Autodesk Inventor part; units mm, degrees
ref_plane "to_cp1_XY" through (0, 0, 0) normal (1, 0, 0) x (0, 0, -1)
ref_plane "to_cp1_YZ" through (0, 0, 0) normal (0, 0, -1) x (0, 1, 0)
ref_plane "to_cp1_ZX" through (0, 0, 0) normal (0, 1, 0) x (1, 0, 0)
sketch "Sketch_1" plane through (0, 0, 0) normal (0, 0, 1) x (1, 0, 0)
  line L0 (50, 0) -> (-50, 0)
  line L1 (0, 12.55) -> (0.33, 12.55)
  line L2 (0.33, 12.55) -> (0.33, 9.2)
  line L3 (0.33, 9.2) -> (0, 9.2)
  line L4 (0, 9.2) -> (0, 7.5)
  line L5 (0, 7.5) -> (7, 7.5)
  line L6 (7, 7.5) -> (7, 9.2)
  line L7 (7, 9.2) -> (6.67, 9.2)
  line L8 (6.67, 9.2) -> (6.67, 12.55)
  line L9 (6.67, 12.55) -> (7, 12.55)
  line L10 (7, 12.55) -> (7, 14)
  line L11 (7, 14) -> (0, 14)
  line L12 (0, 14) -> (0, 12.55)
revolve "Revolution1" add sketch "Sketch_1" angle 360 about axis through (50, 0, 0) along (1, 0, 0)
ref_plane "to_cp1_XY" through (0, 0, 0) normal (1, 0, 0) x (0, 0, -1)
ref_plane "to_cp1_YZ" through (0, 0, 0) normal (0, 0, -1) x (0, 1, 0)
ref_plane "to_cp1_ZX" through (0, 0, 0) normal (0, 1, 0) x (1, 0, 0)
properties part number "C6902ZZ"
Model file for the job. Use its own axes, mm. A direction names the side the tool comes from. Coordinates: 2 decimals unless noted, no trailing zeros. Loops run counter-clockwise (first coordinate to the right, second up) from the corner with the lowest first, then second, coordinate; pieces in that order, holes last. Notation, with made-up numbers: (6, 0.25) - (46, 0.25) arc R9 cw to (46, 14.25) - close; hole circle Ø1 at (-30.75, 83). An arc over 180 degrees is marked (long way). Answer as a JSON object with one key per item and string values. Group by question number.
(1) Cut at A-A (y = 0). Give the cut face in (x, z).
(2) Flat gauge pins, fed straight in: pin 1 (1.5 mm diameter, centred on x = 4, y = 9.5, fed in from -Z); pin 2 (2 mm diameter, centred on x = 4, y = 9, fed in from -Z); pin 3 (3 mm diameter, centred on x = 4, y = -10, fed in from -Z); pin 4 (8 mm diameter, centred on y = -2.5, z = -10.5, fed in from -X). Where does each tip first touch, or does it go through?
(3) Probe line 1 along Z through (x, y) = (6.9, 0); line 2 along Z through (x, y) = (4, 0); line 3 along X through (y, z) = (-11.5, 2.5). List the from-to ranges inside material, lowest first.
(4) Two-plate mould, pull along Y, no slides. Class faces 4 (the face through (0.33, -7, 7)), 5 (the face through (3.451, 12.932, 5.362)), 6 (the face through (7, -8, 0)): released by +Y, released by -Y, zero draft, split by the parting line, or undercut.
(5) Cut at D-D (y = -11.5). Give the cut face in (x, z).
(6) Cut at C-C (x = 5.25). Give the cut face in (y, z), then the cut area to 3 significant figures.
(7) Tool access for faces 1 (the face through (0, -8, 0)), 2 (the face through (6.84, 11.59, -4.81)), 3 (the face through (0.17, 11.59, -4.81)): list every direction of +Z, -Z, +X, -X, +Y, -Y with a clear straight run to the whole face (end or side of a thin tool).
Geometry says:
{
 "1": {"outline": "(0, -14) - (7, -14) - (7, -12.55) - (6.67, -12.55) - (6.67, -9.2) - (7, -9.2) - (7, -7.5) - (0, -7.5) - (0, -9.2) - (0.33, -9.2) - (0.33, -12.55) - (0, -12.55) - close; (0, 7.5) - (7, 7.5) - (7, 9.2) - (6.67, 9.2) - (6.67, 12.55) - (7, 12.55) - (7, 14) - (0, 14) - (0, 12.55) - (0.33, 12.55) - (0.33, 9.2) - (0, 9.2) - close"},
 "2": {"pin 1": "stops at z = -10.93", "pin 2": "stops at z = -11.49", "pin 3": "stops at z = -11.12", "pin 4": "stops at x = 0"},
 "3": {"line 1": "z = -14 to -12.55, -9.2 to -7.5, 7.5 to 9.2, 12.55 to 14", "line 2": "z = -14 to -7.5, 7.5 to 14", "line 3": "x = 0.33 to 6.67"},
 "4": {"face 4": "undercut", "face 5": "split by the parting line", "face 6": "zero draft"},
 "5": {"outline": "(0, -7.98) - (7, -7.98) - (7, -5.03) - (6.67, -5.03) - (6.67, 5.03) - (7, 5.03) - (7, 7.98) - (0, 7.98) - (0, 5.03) - (0.33, 5.03) - (0.33, -5.03) - (0, -5.03) - close"},
 "6": {"outline": "circle Ø28 at (0, 0); hole circle Ø15 at (0, 0)", "area": "439 mm^2"},
 "7": {"face 1": "+Z, -Z, -X, +Y, -Y", "face 2": "+X", "face 3": "-X"}
}
